The listing builds one solid part. Answer for the finished solid, in the listing's coordinates (mm). Face numbers are marked on the shaded views. A direction names the side the tool comes from. Give positions to 0.01 mm unless a question says otherwise; leave off trailing zeros. Loops run counter-clockwise (first coordinate to the right, second up) from the corner with the lowest first, then second, coordinate; pieces in that order, holes last. Notation, with made-up numbers: M 10.25,16.25 L 18.25,16.25 A29 ccw 18.25,49.25 Z; hole C 60.5,87 d6. An arc over 180 degrees is marked long. One line per item, written item: value. Start each with the question number.
Q1. Consider L1, parallel to X at y = -11, z = -8 (3 decimals); L2, parallel to Z at x = -14, y = -25 (3 decimals). Determine where each line is inside the solid, lowest interval first.
Q2. A cutting plane is placed at C-C, the plane x = 11. Determine the outline of the cut face in (y, z) (3 decimals), and give its area (3 significant figures).
Q3. For the marked faces 1 and 2, determine the directions among +Z, -Z, +X, -X, +Y, -Y from which every point of the face is accessible in a straight line to the end or side of a thin tool.
Q4. A cutting plane is placed at B-B, the plane y = 22. Determine the outline of the cut face in (x, z) (3 decimals).
Q5. A flat-ended cylindrical pin translates along its axis: pin 1 (12 mm diameter, centred on x = 26.5, y = 20.5, fed in from -Z). Find the tip coordinate at first contact, or state that the pin passes through.
Q6. A cutting plane is placed at A-A, the plane z = -53.5. Determine the outline of the cut face in (x, y) (3 decimals), and give its area (3 significant figures).
Q7. A cutting plane is placed at D-D, the plane x = 0. Determine the outline of the cut face in (y, z) (3 decimals), and give its area (3 significant figures).
from build123d import *

# Parameters (mm, degrees)
F0_W     = 3.175
F0_H     = 66.04
F1_DEPTH = 3.175
F2_DEPTH = 66.04
F3_R     = 5.08


with BuildPart() as f1:
    # F0 (on Top) → F1 (new body)
    with BuildSketch(Plane.XY):
        with Locations((42.8625, 0)):
            Rectangle(F0_W, F0_H)
        with Locations((-42.8625, 0)):
            Rectangle(F0_W, F0_H)
        with BuildLine():
            Line((41.275, -33.02), (41.275, 33.02))
            Line((41.275, 33.02), (3.81, 33.02))
            ThreePointArc((3.81, 33.02), (0, 29.21), (-3.81, 33.02))
            Line((-3.81, 33.02), (-41.275, 33.02))
            Line((-41.275, 33.02), (-41.275, -33.02))
            Line((-41.275, -33.02), (41.275, -33.02))
        make_face()
    extrude(amount=F1_DEPTH)

    # F0 (on Top) → F2 (join)
    with BuildSketch(Plane.XY):
        with Locations((-42.8625, 0)):
            Rectangle(F0_W, F0_H)
        with Locations((42.8625, 0)):
            Rectangle(F0_W, F0_H)
    extrude(amount=-F2_DEPTH)

    # F3
    f3_edges = [f1.edges().sort_by_distance(p)[0] for p in [
        (-44.45, 0, 3.175),
        (44.45, 0, 3.175),
    ]]
    fillet(f3_edges, radius=F3_R)


solid = f1.part
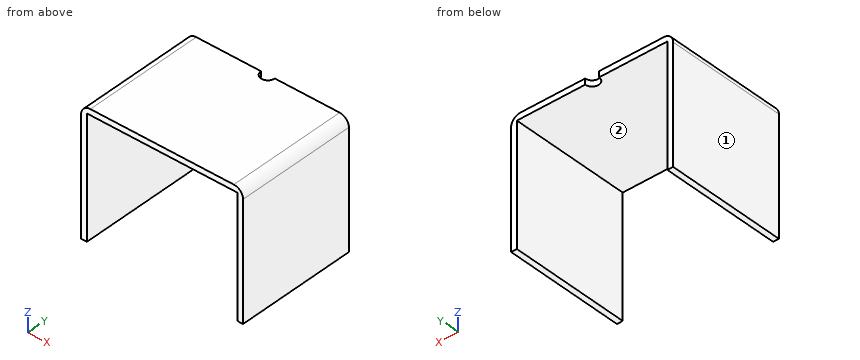
Answer block:
1. L1: -44.45 to -41.275, 41.275 to 44.45
1. L2: 0 to 3.175
2. outline: M -33.02,0 L 33.02,0 L 33.02,3.175 L -33.02,3.175 Z
2. area: 210 mm^2
3. face 1: +Z, -Z, -X, +Y, -Y
3. face 2: -Z, +Y, -Y
4. outline: M -44.45,-66.04 L -41.275,-66.04 L -41.275,0 L 41.275,0 L 41.275,-66.04 L 44.45,-66.04 L 44.45,-1.905 A5.08 ccw 39.37,3.175 L -39.37,3.175 A5.08 ccw -44.45,-1.905 Z
5. pin 1: z = 0
6. outline: M -44.45,-33.02 L -41.275,-33.02 L -41.275,33.02 L -44.45,33.02 Z; M 41.275,-33.02 L 44.45,-33.02 L 44.45,33.02 L 41.275,33.02 Z
6. area: 419 mm^2
7. outline: M -33.02,0 L 29.21,0 L 29.21,3.175 L -33.02,3.175 Z
7. area: 198 mm^2
